from build123d import *

# Parameters (mm, degrees)
REVOLUTION_ANGLE = -180
GROOVE_ANGLE     = -180


with BuildPart() as part:
    # Sketch → Revolution (revolve)
    with BuildSketch(Plane.YZ):
        Polygon((0, 3), (-8.5, 3), (-8.5, 4), (-23.5, 4), (-23.5, -4), (-8.5, -4), (-8.5, -3), (0, -3), align=None)
    revolve(axis=Axis((0, 0, 0), (0, 0, 1)), revolution_arc=REVOLUTION_ANGLE)

    # Import → Groove (revolve, cut)
    with BuildSketch(Plane(origin=(0, -11.25, 0), x_dir=(0, -1, 0), z_dir=(1, 0, 0))):
        Polygon((-11.25, -2), (-1.75, -2), (-1.75, -3), (11.25, -3), (11.25, 3), (-1.75, 3), (-1.75, 2), (-11.25, 2), align=None)
    revolve(axis=Axis((0, 0, 0), (0, 0, 1)), revolution_arc=GROOVE_ANGLE, mode=Mode.SUBTRACT)

    # Sketch002 (on Face3 of Groove) → AdditiveLoft section 0
    with BuildSketch(Plane.YZ):
        Polygon((-23.5, 4), (-8.5, 4), (-8.5, 3), (8.5, 3), (8.5, 4), (23.5, 4), (23.5, -4), (8.5, -4), (8.5, -3), (-8.5, -3), (-8.5, -4), (-23.5, -4), align=None)
    # Import001 → AdditiveLoft section 1
    with BuildSketch(Plane(origin=(92.5, 0, 0), x_dir=(0, 1, 0), z_dir=(-1, 0, 0))):
        Polygon((-28.5, -4), (-13.5, -4), (-13.5, -3), (13.5, -3), (13.5, -4), (28.5, -4), (28.5, 4), (13.5, 4), (13.5, 3), (-13.5, 3), (-13.5, 4), (-28.5, 4), align=None)
    loft()

    # Import002 → SubtractiveLoft section 0
    with BuildSketch(Plane(origin=(0, 0, 0), x_dir=(0, -1, 0), z_dir=(1, 0, 0))):
        Polygon((22.5, -3), (9.5, -3), (9.5, -2), (-9.5, -2), (-9.5, -3), (-22.5, -3), (-22.5, 3), (-9.5, 3), (-9.5, 2), (9.5, 2), (9.5, 3), (22.5, 3), align=None)
    # Import003 → SubtractiveLoft section 1
    with BuildSketch(Plane(origin=(92.5, 0, 0), x_dir=(0, 1, 0), z_dir=(-1, 0, 0))):
        Polygon((-27.5, -3), (-14.5, -3), (-14.5, -2), (14.5, -2), (14.5, -3), (27.5, -3), (27.5, 3), (14.5, 3), (14.5, 2), (-14.5, 2), (-14.5, 3), (-27.5, 3), align=None)
    loft(mode=Mode.SUBTRACT)


solid = part.part
The listing builds one solid part. Answer for the finished solid, in the listing's coordinates (mm). A direction names the side the tool comes from. Coordinates: 2 decimals unless noted, no trailing zeros. Loops run counter-clockwise (first coordinate to the right, second up) from the corner with the lowest first, then second, coordinate; pieces in that order, holes last. Notation, with made-up numbers: (-32, -10.5) -> (16, -10.5) arc R12 cw to (16, 11.5) -> close; hole circle Ø9 at (26, -2). An arc over 180 degrees is marked (long way). Write item = value, one per line. Start each with the question number.
1) A cutting plane is placed at D-D (y = 7). Give the vertices of the cut face in (x, z).
2) Given pin 1 Ø21.5 at (x, y) = (56.5, -2.5) entering from -Z; pin 2 Ø2 at (x, z) = (29.5, 1.5) entering from +Y; pin 3 Ø3 at (x, y) = (44, -3) entering from +Z; pin 4 Ø4 at (x, z) = (62.5, 0) entering from -Y, each flat-ended and moving along its own axis, determine where each tip first touches the part or whether it passes through.
3) Straight lines are drawn through the part: line 1 (Z direction, x = 25, y = 18); line 2 (Z direction, x = 49, y = -6.5); line 3 (Y direction, x = 77.5, z = 2.25). For each, find the intervals that lie inside material, in ascending order. Write a range as from..to.
4) The mould has two halves that part along Y. Classify faces 4 (the face through (-23.494, -0.517, -0.056)), 5 (the face through (46.898, -26.035, -0.056)), 6 (the face through (-8.498, -0.187, -3.493)), 7 (the face through (37, 15, 4)): released by +Y, released by -Y, zero draft, split by the parting line, or undercut.
5) A cutting plane is placed at A-A (z = 0.25). Give the vertices of the cut face in (x, y).
6) A cutting plane is placed at B-B (y = 25.5). Give the vertices of the cut face in (x, z), then the cut area to 3 significant figures.
7) A tool of negligible diameter and unlimited length cuts with its end or side. For faces 1 (the face through (46.898, 12.035, -2.507)), 2 (the face through (46.898, 25.035, 0.042)), 3 (the face through (43, 0, 3)), from which of +Z, -Z, +X, -X, +Y, -Y can it reach the whole face along a straight path? Write none if from no direction.
8) A cutting plane is placed at C-C (x = 67). Give the vertices of the cut face in (y, z).
Responses:
q1.outline = (-22.43, -4) -> (-4.82, -4) -> (-4.82, -3) -> (92.5, -3) -> (92.5, -2) -> (-6.42, -2) -> (-6.42, -3) -> (-21.38, -3) -> (-21.38, 3) -> (-6.42, 3) -> (-6.42, 2) -> (92.5, 2) -> (92.5, 3) -> (-4.82, 3) -> (-4.82, 4) -> (-22.43, 4) -> close
q2.pin_1 = -4
q2.pin_2 = 25.15
q2.pin_3 = 3
q2.pin_4 = -26.99
q3.line_1 = -4..-3, 3..4
q3.line_2 = -3..-2, 2..3
q3.line_3 = -27.69..-26.69, -13.69..13.69, 26.69..27.69
q4.face_4 = split by the parting line
q4.face_5 = released by -Y
q4.face_6 = undercut
q4.face_7 = zero draft
q5.outline = (0, -23.5) -> (92.5, -28.5) -> (92.5, -27.5) -> (0, -22.5) arc R22.5 cw to (0, 22.5) -> (92.5, 27.5) -> (92.5, 28.5) -> (0, 23.5) arc R23.5 ccw to start
q6.outline = (37, -4) -> (92.5, -4) -> (92.5, -3) -> (55.5, -3) -> (55.5, 3) -> (92.5, 3) -> (92.5, 4) -> (37, 4) -> close
q6.area = 222 mm²
q7.face_1 = none
q7.face_2 = +X
q7.face_3 = +Z, +X
q8.outline = (-27.12, -4) -> (-12.12, -4) -> (-12.12, -3) -> (12.12, -3) -> (12.12, -4) -> (27.12, -4) -> (27.12, 4) -> (12.12, 4) -> (12.12, 3) -> (-12.12, 3) -> (-12.12, 4) -> (-27.12, 4) -> close; hole (-26.12, -3) -> (-13.12, -3) -> (-13.12, -2) -> (13.12, -2) -> (13.12, -3) -> (26.12, -3) -> (26.12, 3) -> (13.12, 3) -> (13.12, 2) -> (-13.12, 2) -> (-13.12, 3) -> (-26.12, 3) -> close
